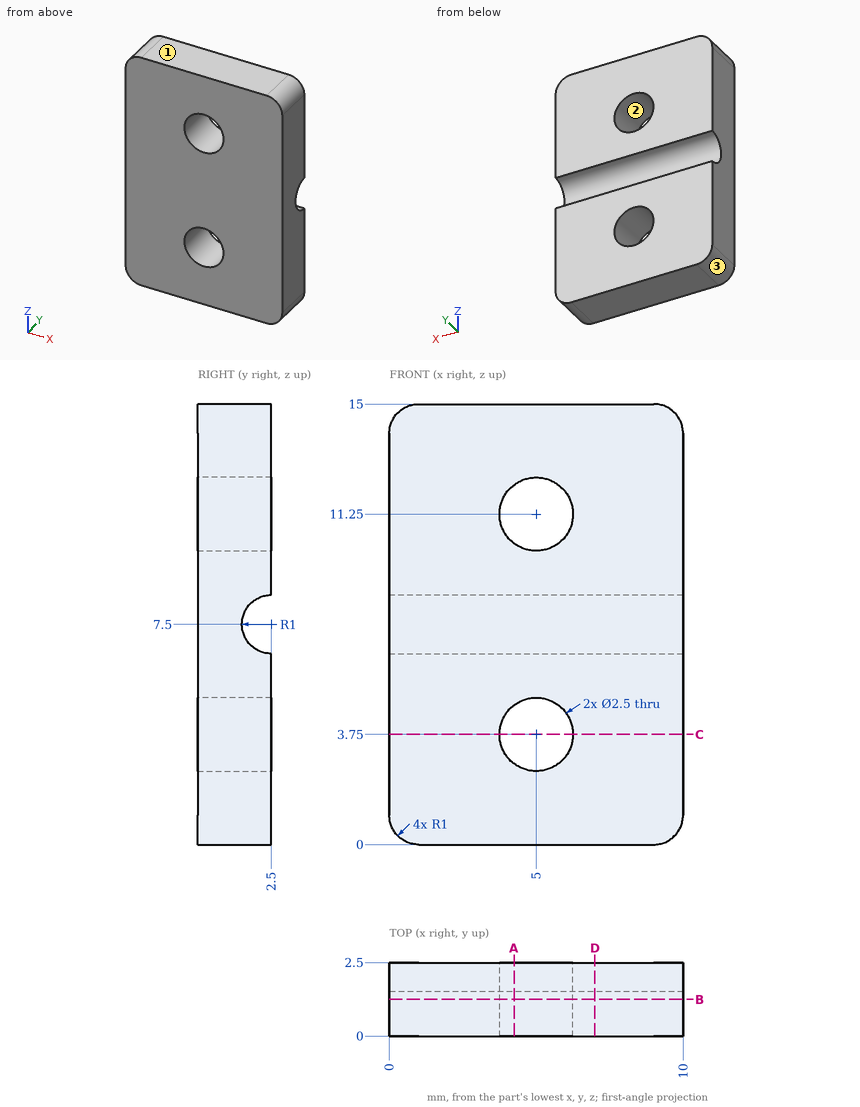
Check sheet for the drawn part. Datum: minimum x, y, z corner. Units: mm. Coordinates: 2 decimals unless noted, no trailing zeros. Write each loop counter-clockwise with the first axis right and the second up, starting at its lowest first coordinate (ties: lowest second). Pieces come first, ordered by that corner, then holes. Notation, with made-up numbers: M 80,52 L 98,52 A34 cw 98,85 Z; hole C 30,35 d10. An arc over 180 degrees is marked long. One line per item, written item: value.
Item 1: Section check D-D, the plane x = 7. Record the boundary of the cut face in (y, z), plus the area to 3 significant figures.
Check sheet entries:
outline: M 0,0 L 2.5,0 L 2.5,6.5 A1 cw 2.5,8.5 L 2.5,15 L 0,15 Z
area: 35.9 mm^2
Item 2: Mould release check, pull along Z, two halves, no side actions. Record for the marked faces 1, 2 and 3: pulls with the +Z half, pulls with the -Z half, needs draft (parallel to the pull), parting line crosses it, or undercut.
Check sheet entries:
face 1: pulls with the +Z half
face 2: undercut
face 3: pulls with the -Z half
Item 3: Scan lines: line 1 along X through (y, z) = (0.75, 3.75); line 2 along Z through (x, y) = (4.25, 0.2); line 3 along Z through (x, y) = (5.5, 0.2). Record each from-to range of solid material in increasing order.
Check sheet entries:
line 1: x = 0 to 3.75, 6.25 to 10
line 2: z = 0 to 2.75, 4.75 to 10.25, 12.25 to 15
line 3: z = 0 to 2.6, 4.9 to 10.1, 12.4 to 15
Item 4: Section check C-C, the plane z = 3.75. Record the boundary of the cut face in (x, y).
Check sheet entries:
outline: M 0,0 L 3.75,0 L 3.75,2.5 L 0,2.5 Z; M 6.25,0 L 10,0 L 10,2.5 L 6.25,2.5 Z
Item 5: Section check A-A, the plane x = 4.25. Record the boundary of the cut face in (y, z).
Check sheet entries:
outline: M 0,0 L 2.5,0 L 2.5,2.75 L 0,2.75 Z; M 0,4.75 L 2.5,4.75 L 2.5,6.5 A1 cw 2.5,8.5 L 2.5,10.25 L 0,10.25 Z; M 0,12.25 L 2.5,12.25 L 2.5,15 L 0,15 Z
Item 6: Section check B-B, the plane y = 1.25. Record the boundary of the cut face in (x, z).
Check sheet entries:
outline: M 0,1 A1 ccw 1,0 L 9,0 A1 ccw 10,1 L 10,14 A1 ccw 9,15 L 1,15 A1 ccw 0,14 Z; hole C 5,3.75 d2.5; hole C 5,11.25 d2.5
